Input: part model. Units: mm. Frame: model coordinates. Give positions to 0.01 mm unless a question says otherwise; leave off trailing zeros. Loops run counter-clockwise (first coordinate to the right, second up) from the corner with the lowest first, then second, coordinate; pieces in that order, holes last. Notation, with made-up numbers: (44.5, 33) -> (68.5, 33) arc R24 cw to (68.5, 48) -> close; hole circle Ø11 at (76.25, 70). An arc over 180 degrees is marked (long way). Answer as a JSON object with one key per item and string values.
```python
from build123d import *

# Parameters (mm, degrees)
F0_W           = 320
F0_H           = 260
F1_DEPTH       = 2.5
F3_D           = 4.4
F3_DEPTH       = 17.25
F3_CSINK_D     = 8.96
F3_CSINK_ANGLE = 90
F3_TIP         = 1.3218933619
F5_D           = 8.8
F5_DEPTH       = 17.25
F5_TIP         = 2.6437867237
F7_D           = 4.4
F7_DEPTH       = 17.25
F7_TIP         = 1.3218933619
F9_D           = 22
F9_DEPTH       = 17.25
F9_TIP         = 6.6094668093
F10_W          = 13
F10_H          = 28
F11_DEPTH      = 25


# Not quite as in the source:
# - a feature names something its author has since deleted; it is built from what else it names


with BuildPart() as f1:
    # F0 (on Top) → F1 (new body, symmetric)
    with BuildSketch(Plane.XY):
        Rectangle(F0_W, F0_H)
    extrude(amount=F1_DEPTH, both=True)

    # F3
    with Locations(Plane.XY.offset(2.5)):
        with Locations((-155, -96), (-155, 124), (155, 124), (155, -96)):
            CounterSinkHole(F3_D / 2, F3_CSINK_D / 2, depth=F3_DEPTH, counter_sink_angle=F3_CSINK_ANGLE)
            with Locations((0, 0, -(F3_DEPTH + F3_TIP / 2))):  # 118° drill point
                Cone(0, F3_D / 2, F3_TIP, mode=Mode.SUBTRACT)

    # F5
    with Locations(Plane.XY.offset(2.5)):
        with Locations((-62.5, 115), (-62.5, 100), (-40.5, 115), (-40.5, 100), (-18.5, 115), (3.5, 100), (3.5, 115), (-18.5, 100), (25.5, 100), (25.5, 115), (47.5, 115), (69.5, 115), (91.5, 115), (91.5, 100), (113.5, 100), (113.5, 115), (47.5, 100), (69.5, 100), (135.5, 115), (135.5, 100)):
            Hole(F5_D / 2, depth=F5_DEPTH)
            with Locations((0, 0, -(F5_DEPTH + F5_TIP / 2))):  # 118° drill point
                Cone(0, F5_D / 2, F5_TIP, mode=Mode.SUBTRACT)

    # F7
    with Locations(Plane.XY.offset(2.5)):
        with Locations((-99, 50), (-99, -10), (-99, -70), (-33, -70), (-33, -10), (-33, 50), (33, 50), (99, 50), (99, -10), (33, -10), (33, -70), (99, -70)):
            Hole(F7_D / 2, depth=F7_DEPTH)
            with Locations((0, 0, -(F7_DEPTH + F7_TIP / 2))):  # 118° drill point
                Cone(0, F7_D / 2, F7_TIP, mode=Mode.SUBTRACT)

    # F9
    with Locations(Plane.XY.offset(2.5)):
        with Locations((-125, 108), (-125, 73), (-125, 38)):
            Hole(F9_D / 2, depth=F9_DEPTH)
            with Locations((0, 0, -(F9_DEPTH + F9_TIP / 2))):  # 118° drill point
                Cone(0, F9_D / 2, F9_TIP, mode=Mode.SUBTRACT)

    # F10 (on face) → F11 (cut)
    with BuildSketch(Plane.XY.offset(2.5)):
        with Locations((-90.5, 107.5)):
            Rectangle(F10_W, F10_H)
    extrude(amount=-F11_DEPTH, mode=Mode.SUBTRACT)


solid = f1.part
```
Q1. Section C-C, the plane z = -1.05. Give the number of separate pieces and of enclosed holes in the cut face, then the cut area to 3 significant figures.
Evaluation:
{"separate pieces": "1", "enclosed holes": "40", "area": "80,200 mm2"}
Q2. Ray query, line 1 along Y through (x, z) = (47.5, 0.35); line 2 along X through (y, z) = (-96, -0.7); line 3 along Y through (x, z) = (-33, 0.95). Return the intervals inside material, ascending.
Evaluation:
{"line 1": "y = -130 to 95.6, 104.4 to 110.6, 119.4 to 130", "line 2": "x = -160 to -157.2, -152.8 to 152.8, 157.2 to 160", "line 3": "y = -130 to -72.2, -67.8 to -12.2, -7.8 to 47.8, 52.2 to 130"}
Q3. Section B-B, the plane x = -130. Return the cut outline in (y, z), then the cut area to 3 significant figures.
Evaluation:
{"outline": "(-130, -2.5) -> (28.2, -2.5) -> (28.2, 2.5) -> (-130, 2.5) -> close; (47.8, -2.5) -> (63.2, -2.5) -> (63.2, 2.5) -> (47.8, 2.5) -> close; (82.8, -2.5) -> (98.2, -2.5) -> (98.2, 2.5) -> (82.8, 2.5) -> close; (117.8, -2.5) -> (130, -2.5) -> (130, 2.5) -> (117.8, 2.5) -> close", "area": "1,010 mm2"}
Q4. Section A-A, the plane y = 38. Return the cut outline in (x, z).
Evaluation:
{"outline": "(-160, -2.5) -> (-136, -2.5) -> (-136, 2.5) -> (-160, 2.5) -> close; (-114, -2.5) -> (160, -2.5) -> (160, 2.5) -> (-114, 2.5) -> close"}
